Verification items for the finished model (mm, model axes). A direction names the side the tool comes from. Give positions to 0.01 mm unless a question says otherwise; leave off trailing zeros. Loops run counter-clockwise (first coordinate to the right, second up) from the corner with the lowest first, then second, coordinate; pieces in that order, holes last. Notation, with made-up numbers: (25.5, -18.5) -> (58.5, -18.5) arc R21 cw to (58.5, -0.5) -> close; hole circle Ø8 at (-36.5, 28.25). An arc over 180 degrees is marked (long way). Answer in a Markdown table with one row per item. Add a question column.
Q1. Section check B-B on x = 28.75. Enter the section's corners in (y, z), and give its area (3 significant figures).
Q2. Material ranges on probe 1 along X at (y, z) = (7.5, -0.5); probe 2 along Z at (x, y) = (33, 7.75); probe 3 along Y at (x, z) = (-8.25, -1.8), recorded low to high.
Q3. Section check D-D on x = 0. Enter the section's corners in (y, z).
Q4. Release check for a two-part mould opening along X. For faces 1 (the face through (26.6, 5.1, 2.1)), 2 (the face through (1, 5, 6)), 3 (the face through (39, 5, 0)) record: pulls with the +X half, pulls with the -X half, needs draft (parallel to the pull), parting line crosses it, or undercut.
Q5. Gauge pin test, flat ends, axial feed: P1, Ø5, axis at x = 30, y = 5.5, coming from the +Z side; P2, Ø2.5, axis at x = -8.25, y = 5, coming from the -Z side; P3, Ø3, axis at x = -15, y = 2.5, coming from the -Z side; P4, Ø2, axis at x = 3, y = 2, coming from the -Z side. Record the tip position at first contact, or that the pin passes through.
Q6. Set-up check for faces 4 (the face through (-24, 5, -6)), 5 (the face through (-4.292, 2.465, -26.475)), 6 (the face through (9.5, 5, -18)), 7 (the face through (27.44, 4, -0.46)): record each of +Z, -Z, +X, -X, +Y, -Y from which the full face is reachable in a straight line by a thin tool's end or side.
Q7. Section check C-C on y = 8.5. Enter the section's corners in (x, z), and give its area (3 significant figures).
Q8. Section check A-A on z = -0.5. Enter the section's corners in (x, y).
```python
from build123d import *

# Parameters (mm, degrees)
IZIM1_R                     = 3.25
IZIM1_R_2                   = 2.25
Y_KSEKLIK_EKSTR_ZYON1_DEPTH = 10
KES_EKSTR_ZYON1_DEPTH       = 5
IZIM3_R                     = 2
KES_EKSTR_ZYON4_DEPTH       = 4
IZIM4_W                     = 6.1
IZIM4_H                     = 2.8
IZIM4_W_2                   = 6
KES_EKSTR_ZYON5_DEPTH       = 10
IZIM5_R                     = 1.65
KES_EKSTR_ZYON6_DEPTH       = 5
IZIM6_R                     = 2
KES_EKSTR_ZYON7_DEPTH       = 13


with BuildPart() as part:
    # Çizim1 → Yükseklik-Ekstrüzyon1 (new body)
    with BuildSketch(Plane(origin=(0, 0, 0), x_dir=(1, 0, 0), z_dir=(0, 1, 0))):
        with BuildLine():
            Line((9.5, 6), (39, 6))
            Line((39, 6), (39, -6))
            Line((39, -6), (-39, -6))
            Line((-39, -6), (-39, 6))
            Line((-39, 6), (-9.5, 6))
            Line((-9.5, 6), (-9.5, 29))
            ThreePointArc((-9.5, 29), (0, 38.5), (9.5, 29))
            Line((9.5, 29), (9.5, 6))
        make_face()
        with Locations(Location((0, 29, 0), (0, 0, 270))):
            Circle(IZIM1_R, mode=Mode.SUBTRACT)
        with Locations(Location((-33, 0.5, 0), (0, 0, 270))):
            Circle(IZIM1_R_2, mode=Mode.SUBTRACT)
        with Locations(Location((33, 0.5, 0), (0, 0, 90))):
            Circle(IZIM1_R_2, mode=Mode.SUBTRACT)
    extrude(amount=Y_KSEKLIK_EKSTR_ZYON1_DEPTH)

    # Çizim2 → Kes-Ekstrüzyon1 (cut)
    with BuildSketch(Plane.XZ):
        Polygon((5.75, -29), (2.875, -24.020353928), (-2.875, -24.020353928), (-5.75, -29), (-2.875, -33.979646072), (2.875, -33.979646072), align=None)
    extrude(amount=-KES_EKSTR_ZYON1_DEPTH, mode=Mode.SUBTRACT)

    # Çizim3 → Kes-Ekstrüzyon4 (cut)
    with BuildSketch(Plane.XY.offset(6)):
        with Locations((-8.25, 5)):
            Circle(IZIM3_R)
        with Locations((28.75, 5)):
            Circle(IZIM3_R)
    extrude(amount=-KES_EKSTR_ZYON4_DEPTH, mode=Mode.SUBTRACT)

    # Çizim4 → Kes-Ekstrüzyon5 (cut)
    with BuildSketch(Plane(origin=(0, 10, 0), x_dir=(1, 0, 0), z_dir=(0, 1, 0))):
        with Locations((-8.380873527, -3.5)):
            Rectangle(IZIM4_W, IZIM4_H)
        with Locations((28.619126473, -3.5)):
            Rectangle(IZIM4_W_2, IZIM4_H)
    extrude(amount=-KES_EKSTR_ZYON5_DEPTH, mode=Mode.SUBTRACT)

    # Çizim5 → Kes-Ekstrüzyon6 (cut)
    with BuildSketch(Plane.XY.offset(2)):
        with Locations((-8.25, 5)):
            Circle(IZIM5_R)
        with Locations((28.75, 5)):
            Circle(IZIM5_R)
    extrude(amount=-KES_EKSTR_ZYON6_DEPTH, mode=Mode.SUBTRACT)

    # Çizim6 → Kes-Ekstrüzyon7 (cut)
    with BuildSketch(Plane(origin=(0, 10, 0), x_dir=(1, 0, 0), z_dir=(0, 1, 0))):
        with Locations(Location((-20, 0.5, 0), (0, 0, 270))):
            Circle(IZIM6_R)
        with Locations(Location((20, 0.5, 0), (0, 0, 270))):
            Circle(IZIM6_R)
    extrude(amount=-KES_EKSTR_ZYON7_DEPTH, mode=Mode.SUBTRACT)


solid = part.part
```
Taken from the geometry:
| question | item | result |
|---|---|---|
| 1 | outline | (0, -6) -> (10, -6) -> (10, 2.1) -> (7, 2.1) -> (7, 2) -> (6.65, 2) -> (6.65, -3) -> (3.35, -3) -> (3.35, 2) -> (3, 2) -> (3, 2.1) -> (0, 2.1) -> close; (0, 4.9) -> (3, 4.9) -> (3, 6) -> (0, 6) -> close; (7, 4.9) -> (10, 4.9) -> (10, 6) -> (7, 6) -> close |
| 1 | area | 70.7 mm² |
| 2 | probe 1 | x = -39 to -35.25, -30.75 to -22, -18 to 18, 22 to 30.75, 35.25 to 39 |
| 2 | probe 2 | z = -6 to -2.75, 1.75 to 6 |
| 2 | probe 3 | y = 0 to 3.35, 6.65 to 10 |
| 3 | outline | (0, -38.5) -> (10, -38.5) -> (10, -32.25) -> (5, -32.25) -> (5, -33.98) -> (0, -33.98) -> close; (0, -24.02) -> (5, -24.02) -> (5, -25.75) -> (10, -25.75) -> (10, 6) -> (0, 6) -> close |
| 4 | face 1 | undercut |
| 4 | face 2 | needs draft |
| 4 | face 3 | pulls with the +X half |
| 5 | P1 | stops at z = 6 |
| 5 | P2 | stops at z = -35.42 |
| 5 | P3 | stops at z = -6 |
| 5 | P4 | stops at z = -38.29 |
| 6 | face 4 | -Z, -X, +Y, -Y |
| 6 | face 5 | -Y |
| 6 | face 6 | -Z, +X, +Y, -Y |
| 6 | face 7 | +Z |
| 7 | outline | (-39, -6) -> (-9.5, -6) -> (-9.5, -29) arc R9.5 ccw to (9.5, -29) -> (9.5, -6) -> (39, -6) -> (39, 6) -> (-39, 6) -> close; hole circle Ø4.5 at (-33, -0.5); hole circle Ø4 at (-20, -0.5); hole (-11.43, 2.1) -> (-5.33, 2.1) -> (-5.33, 4.9) -> (-11.43, 4.9) -> close; hole circle Ø6.5 at (0, -29); hole circle Ø4 at (20, -0.5); hole (25.62, 2.1) -> (31.62, 2.1) -> (31.62, 4.9) -> (25.62, 4.9) -> close; hole circle Ø4.5 at (33, -0.5) |
| 7 | area | 1,390 mm² |
| 8 | outline | (-39, 0) -> (-35.25, 0) -> (-35.25, 10) -> (-39, 10) -> close; (-30.75, 0) -> (-22, 0) -> (-22, 10) -> (-30.75, 10) -> close; (-18, 0) -> (18, 0) -> (18, 10) -> (-18, 10) -> close; (22, 0) -> (30.75, 0) -> (30.75, 10) -> (22, 10) -> close; (35.25, 0) -> (39, 0) -> (39, 10) -> (35.25, 10) -> close; hole circle Ø3.3 at (-8.25, 5); hole circle Ø3.3 at (28.75, 5) |
